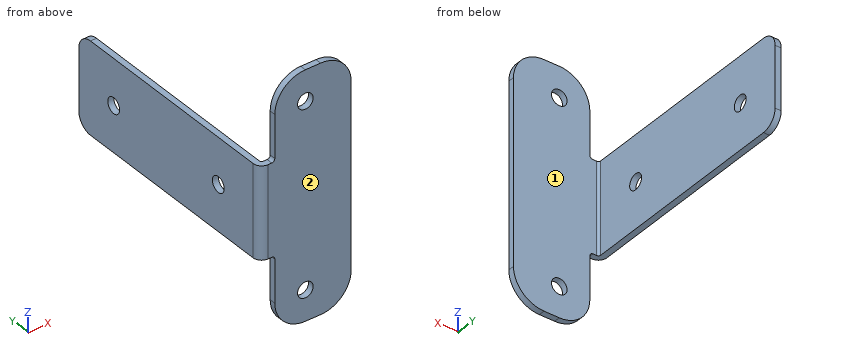
from build123d import *

# Parameters (mm, degrees)
SKETCH1_R                  = 2.55
BASE_FLANGE1_DEPTH         = 2
SKETCHED_START             = -90
SKETCHED_BEND1_OUTLINE_W   = 2
SKETCHED_BEND1_OUTLINE_H   = 30
SKETCHED_BEND1_DEPTH       = 75
SKETCHED_START_2           = -14.733838284
SKETCHED_BEND1_2_OUTLINE_R = 2.55
SKETCHED_BEND1_2_DEPTH     = 1.733838284
SKETCHED_START_3           = -15
SKETCHED_BEND1_3_OUTLINE_R = 2.55
SKETCHED_BEND1_3_DEPTH     = 2.7366
SKETCHED_START_4           = -16
SKETCHED_BEND1_4_DEPTH     = 31


with BuildPart() as part:
    # Base-Flange1: sheet metal written as solids
    # Sketch1 → Base-Flange1 (new body)
    with BuildSketch(Plane(origin=(0, 0, 0), x_dir=(1, 0, 0), z_dir=(0, 1, 0))):
        with BuildLine():
            Line((0, 40), (5, 40))
            ThreePointArc((5, 40), (12.071067812, 37.071067812), (15, 30))
            Line((15, 30), (15, 0))
            Line((15, 0), (15, -30))
            ThreePointArc((15, -30), (12.071067812, -37.071067812), (5, -40))
            Line((5, -40), (0, -40))
            ThreePointArc((0, -40), (-7.071067812, -37.071067812), (-10, -30))
            Line((-10, -30), (-10, -16))
            ThreePointArc((-10, -16), (-10.292893219, -15.292893219), (-11, -15))
            Line((-11, -15), (-20, -15))
            Line((-20, -15), (-85, -15))
            ThreePointArc((-85, -15), (-88.535533906, -13.535533906), (-90, -10))
            Line((-90, -10), (-90, 10))
            ThreePointArc((-90, 10), (-88.535533906, 13.535533906), (-85, 15))
            Line((-85, 15), (-20, 15))
            Line((-20, 15), (-11, 15))
            ThreePointArc((-11, 15), (-10.292893219, 15.292893219), (-10, 16))
            Line((-10, 16), (-10, 30))
            ThreePointArc((-10, 30), (-7.071067812, 37.071067812), (0, 40))
        make_face()
        with Locations(Location((0, -30, 0), (0, 0, 90))):
            Circle(SKETCH1_R, mode=Mode.SUBTRACT)
        with Locations(Location((0, 30, 0), (0, 0, 270))):
            Circle(SKETCH1_R, mode=Mode.SUBTRACT)
        with Locations(Location((-75, 0, 0), (0, 0, 270))):
            Circle(SKETCH1_R, mode=Mode.SUBTRACT)
        with Locations(Location((-30, 0, 0), (0, 0, 270))):
            Circle(SKETCH1_R, mode=Mode.SUBTRACT)
    extrude(amount=-BASE_FLANGE1_DEPTH)

    # Sketched Bend1: read off the stored shape, not the designer's step
    # Sketched Bend1 outline → Sketched Bend1 (cut)
    with BuildSketch(Plane.YZ.offset(SKETCHED_START)):
        with Locations((-1, 0)):
            Rectangle(SKETCHED_BEND1_OUTLINE_W, SKETCHED_BEND1_OUTLINE_H)
    extrude(amount=SKETCHED_BEND1_DEPTH, mode=Mode.SUBTRACT)

    # Sketched Bend1 2 outline → Sketched Bend1 2 (add)
    with BuildSketch(Plane.YZ.offset(SKETCHED_START_2)):
        with BuildLine():
            ThreePointArc((75.745355099, 10), (74.280889005, 13.535533906), (70.745355099, 15))
            Line((70.745355099, 15), (0, 15))
            Line((0, 15), (0, -15))
            Line((0, -15), (70.745355099, -15))
            ThreePointArc((70.745355099, -15), (74.280889005, -13.535533906), (75.745355099, -10))
            Line((75.745355099, -10), (75.745355099, 10))
        make_face()
        with Locations((15.745355099, 0)):
            Circle(SKETCHED_BEND1_2_OUTLINE_R, mode=Mode.SUBTRACT)
        with Locations((60.745355099, 0)):
            Circle(SKETCHED_BEND1_2_OUTLINE_R, mode=Mode.SUBTRACT)
    extrude(amount=SKETCHED_BEND1_2_DEPTH)

    # Sketched Bend1 3 outline → Sketched Bend1 3 (add)
    with BuildSketch(Plane.YZ.offset(SKETCHED_START_3)):
        with BuildLine():
            ThreePointArc((75.745355099, 10), (74.280889005, 13.535533906), (70.745355099, 15))
            Line((70.745355099, 15), (0, 15))
            Line((0, 15), (0, -15))
            Line((0, -15), (70.745355099, -15))
            ThreePointArc((70.745355099, -15), (74.280889005, -13.535533906), (75.745355099, -10))
            Line((75.745355099, -10), (75.745355099, 10))
        make_face()
        with Locations((15.745355099, 0)):
            Circle(SKETCHED_BEND1_3_OUTLINE_R, mode=Mode.SUBTRACT)
        with Locations((60.745355099, 0)):
            Circle(SKETCHED_BEND1_3_OUTLINE_R, mode=Mode.SUBTRACT)
    extrude(amount=SKETCHED_BEND1_3_DEPTH)

    # Sketched Bend1 4 outline → Sketched Bend1 4 (cut)
    with BuildSketch(Plane.XY.offset(SKETCHED_START_4)):
        with BuildLine():
            Line((-12.2634, 75.745355099), (-13, 75.745355099))
            Line((-13, 75.745355099), (-13, 0.7366))
            ThreePointArc((-13, 0.7366), (-12.784254855, 0.215745145), (-12.2634, 0))
            Line((-12.2634, 0), (-12.2634, 75.745355099))
        make_face()
        with BuildLine():
            ThreePointArc((-12.2634, -2), (-14.198468417, -1.198468417), (-15, 0.7366))
            Line((-15, 0.7366), (-15, -2))
            Line((-15, -2), (-12.2634, -2))
        make_face()
    extrude(amount=SKETCHED_BEND1_4_DEPTH, mode=Mode.SUBTRACT)


solid = part.part
Verification items for the finished model (mm, model axes). Face numbers are marked on the shaded views. A direction names the side the tool comes from. Coordinates: 2 decimals unless noted, no trailing zeros. Loops run counter-clockwise (first coordinate to the right, second up) from the corner with the lowest first, then second, coordinate; pieces in that order, holes last. Notation, with made-up numbers: M -34.5,-9.75 L 1.5,-9.75 A20 ccw 1.5,-1.75 Z; hole C 86,76 d3. An arc over 180 degrees is marked long. One line per item, written item: value.
1. Set-up check for the marked faces 1 and 2: record each of +Z, -Z, +X, -X, +Y, -Y from which the full face is reachable in a straight line by a thin tool's end or side.
Answers follow:
face 1: +Z, -Z, +X, +Y
face 2: +Z, -Z, +X, -X, -Y
2. Section check A-A on z = 0. Record the cut outline in (x, y).
Answers follow:
outline: M -15,0.74 A2.74 ccw -12.26,-2 L 15,-2 L 15,0 L -12.26,0 A0.74 cw -13,0.74 L -13,13.2 L -15,13.2 Z; M -15,18.3 L -13,18.3 L -13,58.2 L -15,58.2 Z; M -15,63.3 L -13,63.3 L -13,75.75 L -15,75.75 Z
3. Section check B-B on x = 4. Record the cut outline in (y, z), plus the area to 3 significant figures.
Answers follow:
outline: M -2,-40 L 0,-40 L 0,40 L -2,40 Z
area: 160 mm^2
4. Section check D-D on y = 34. Record the cut outline in (x, z).
Answers follow:
outline: M -15,-15 L -13,-15 L -13,15 L -15,15 Z
5. Section check C-C on z = 12. Record the cut outline in (x, y).
Answers follow:
outline: M -15,0.74 A2.74 ccw -12.26,-2 L 15,-2 L 15,0 L -12.26,0 A0.74 cw -13,0.74 L -13,75.33 L -15,75.33 Z
6. Gauge pin test, flat ends, axial feed: P1, Ø2, axis at x = -4.5, z = 16.5, coming from the +Y side; P2, Ø15, axis at y = 40.5, z = 2.5, coming from the +X side; P3, Ø1.6, axis at y = -1, z = -21.5, coming from the -X side. Record the tip position at first contact, or that the pin passes through.
Answers follow:
P1: y = 0
P2: x = -13
P3: x = -10
7. Material ranges on line 1 along Y through (x, z) = (-14.1, 0); line 2 along Y through (x, z) = (-13.5, 0); line 3 along X through (y, z) = (-0.35, -30), recorded low to high. Write a range as from..to.
Answers follow:
line 1: -1.29..13.2, 18.3..58.2, 63.3..75.75
line 2: -1.7..13.2, 18.3..58.2, 63.3..75.75
line 3: -10..-2.55, 2.55..15
